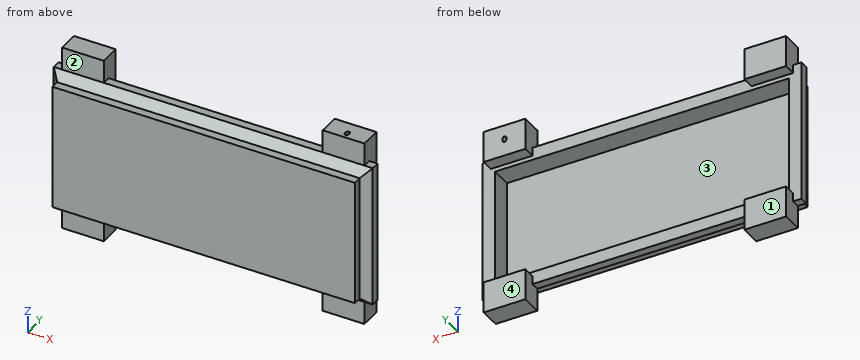
from build123d import *

# Parameters (mm, degrees)
SKETCH1_W               = 145
SKETCH1_H               = 60
SKETCH1_W_2             = 141
SKETCH1_H_2             = 56
BOSS_EXTRUDE1_DEPTH     = 10
SKETCH2_W               = 145
SKETCH2_H               = 60
BOSS_EXTRUDE2_DEPTH     = 2
SKETCH3_W               = 153
SKETCH3_H               = 68
SKETCH3_W_2             = 145
SKETCH3_H_2             = 60
BOSS_EXTRUDE3_DEPTH     = 4
CHAMFER1_SIZE           = 4
BOSS_EXTRUDE4_START     = -4
SKETCH4_W               = 20
SKETCH4_H               = 15
BOSS_EXTRUDE4_DEPTH     = 10
CUT_EXTRUDE2_DEPTH      = 102.600935035
CUT_EXTRUDE2_DEPTH_BACK = 102.600935035
SKETCH6_R               = 1


with BuildPart() as part:
    # Sketch1 → Boss-Extrude1 (new body)
    with BuildSketch(Plane(origin=(0, 0, 0), x_dir=(1, 0, 0), z_dir=(0, 1, 0))):
        Rectangle(SKETCH1_W, SKETCH1_H)
        Rectangle(SKETCH1_W_2, SKETCH1_H_2, mode=Mode.SUBTRACT)
    extrude(amount=BOSS_EXTRUDE1_DEPTH)

    # Sketch2 → Boss-Extrude2 (add)
    with BuildSketch(Plane.XZ):
        Rectangle(SKETCH2_W, SKETCH2_H)
    extrude(amount=BOSS_EXTRUDE2_DEPTH)

    # Sketch3 → Boss-Extrude3 (add)
    with BuildSketch(Plane(origin=(0, 10, 0), x_dir=(1, 0, 0), z_dir=(0, 1, 0))):
        Rectangle(SKETCH3_W, SKETCH3_H)
        Rectangle(SKETCH3_W_2, SKETCH3_H_2, mode=Mode.SUBTRACT)
    extrude(amount=-BOSS_EXTRUDE3_DEPTH)

    # Chamfer1
    chamfer1_edges = [part.edges().sort_by_distance(p)[0] for p in [
        (-72.5, 6, 0),
        (0, 6, 30),
        (72.5, 6, 0),
        (0, 6, -30),
    ]]
    chamfer(chamfer1_edges, length=CHAMFER1_SIZE - 0.0001)  # a hair under: the kernel refuses the full size

    # Sketch4 → Boss-Extrude4 (add)
    with BuildSketch(Plane(origin=(0, 10, 0), x_dir=(1, 0, 0), z_dir=(0, 1, 0)).offset(BOSS_EXTRUDE4_START)):
        with Locations((-62.5, 37.5)):
            Rectangle(SKETCH4_W, SKETCH4_H)
        with Locations((-62.5, -37.5)):
            Rectangle(SKETCH4_W, SKETCH4_H)
        with Locations((62.5, -37.5)):
            Rectangle(SKETCH4_W, SKETCH4_H)
        with Locations((62.5, 37.5)):
            Rectangle(SKETCH4_W, SKETCH4_H)
    extrude(amount=BOSS_EXTRUDE4_DEPTH)

    # Sketch6 → Cut-Extrude2 (cut, two sides: drawn at the far end of the back side and taken through both)
    with BuildSketch(Plane(origin=(0, -14.5, 14.5), x_dir=(1, 0, 0), z_dir=(0, 0.7071067811865464, -0.7071067811865488)).offset(-CUT_EXTRUDE2_DEPTH_BACK)):
        with Locations(Location((62.5, -38.261881076, 0), (0, 0, 270))):
            Circle(SKETCH6_R)
    extrude(amount=CUT_EXTRUDE2_DEPTH + CUT_EXTRUDE2_DEPTH_BACK, mode=Mode.SUBTRACT)


solid = part.part
Build history of the part. All positions in model axes, mm. Face numbers are marked on the shaded views. A direction names the side the tool comes from. Coordinates: 2 decimals unless noted, no trailing zeros. Order: outer loops, then holes, each group sorted by start corner. A loop starts at its lowest first (then second) coordinate and runs counter-clockwise, first axis right, second up. Notation, with made-up numbers: M 75,-6.5 L 124,-6.5 A31 cw 124,30.5 Z; hole C 40,55.25 d4. An arc over 180 degrees is marked long. One line per question, with ' | ' between items. Start each with the question number.
Q1. Probe L1, parallel to Z at x = -56, y = 11.5; L2, parallel to Z at x = -68, y = 0.5; L3, parallel to X at y = 9.75, z = -23.5. List the from-to ranges inside material, lowest first. Write a range as from..to.
Q2. Saw through at A-A (x = 58.5). List the corners of the cut face in (y, z).
Q3. Two-plate mould, pull along X, no slides. Class the marked faces 3 and 4: +X half, -X half, draft (parallel to the pull), parting line (faces both ways), or undercut.
Q4. Saw through at C-C (y = 13.25). Count the separate pieces of the cut face and the enclosed holes in it, then the cut area to 3 significant figures.
Q5. Flat gauge pins, fed straight in: pin 1 Ø5 at (x, y) = (6, 6) entering from -Z; pin 2 Ø8 at (y, z) = (11, -41) entering from +X; pin 3 Ø1 at (x, y) = (-9.5, 1) entering from +Z. Where does each tip first touch, or does it go through?
Q6. 3-axis set-ups, long thin cutter, end or side, ignore diameter. For the marked faces 1 and 2: which of +Z, -Z, +X, -X, +Y, -Y reach the whole face in a straight line?
Check values:
1) L1: z = -45..-30, 30..45 | L2: z = -30..-28, 28..30 | L3: x = -76.5..-70.5, 70.5..76.5
2) outline: M -2,-30 L 2,-30 L 6,-34 L 6,-45 L 16,-45 L 16,-30 L 10,-30 L 10,-28 L 0,-28 L 0,28 L 10,28 L 10,30 L 16,30 L 16,45 L 6,45 L 6,34 L 2,30 L -2,30 Z
3) face 3: undercut | face 4: draft
4) separate pieces: 4 | enclosed holes: 1 | area: 1,200 mm2
5) pin 1: stops at z = -34 | pin 2: stops at x = 72.5 | pin 3: stops at z = 30
6) face 1: +Z, -Z, +X, -X, +Y | face 2: +Z, +X, -X, -Y
